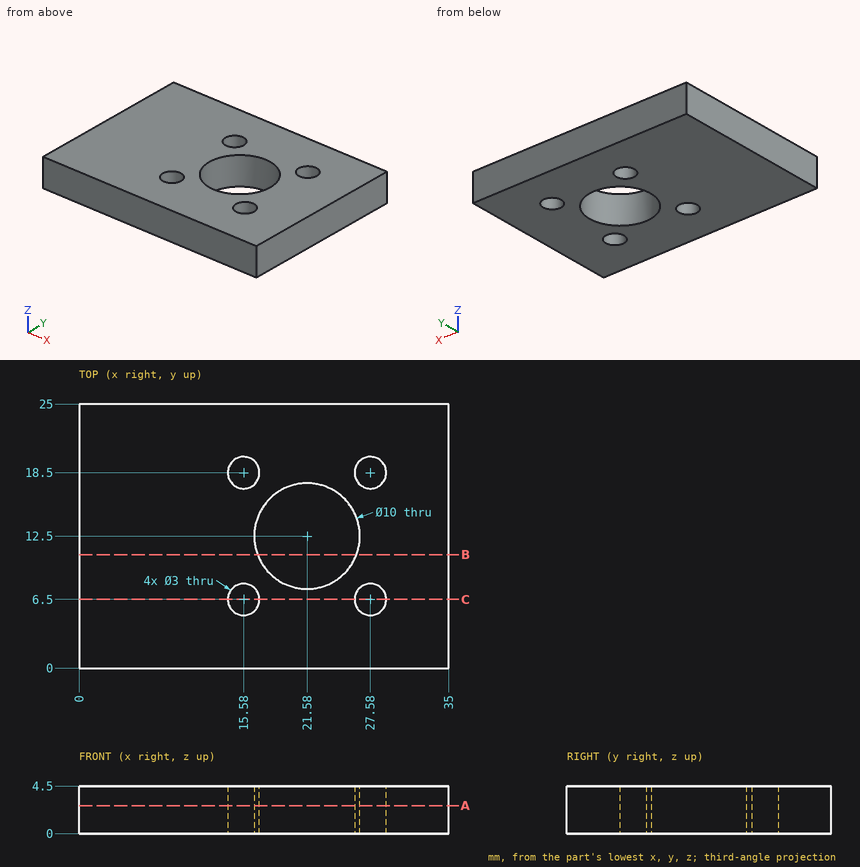
Design review of the part shown in the three views and the two pictorial views. Dimensions are in mm from the part's minimum x, y and z. Coordinates: 2 decimals unless noted, no trailing zeros. Order: outer loops, then holes, each group sorted by start corner. A loop starts at its lowest first (then second) coordinate and runs counter-clockwise, first axis right, second up.
1) Clearance check with a flat-ended pin moving along its axis: pin 1 (1 mm diameter, centred on x = 6.5, z = 3, fed in from -Y). State where the tip first meets the part, or that it passes through.
2) Wall thickness on line 1 along Y through (x, z) = (27.5, 2.7); line 2 along X through (y, z) = (5.25, 0.8); line 3 along X through (y, z) = (21.75, 3.35) (1 decimal): over which ranges is each line inside the solid? List them lowest first.
3) Take a section at B-B, the plane y = 10.75. Give the boundary of the cut face in (x, z), and give its area (3 significant figures).
4) Take a section at C-C, the plane y = 6.5. Give the boundary of the cut face in (x, z).
5) Take a section at A-A, the plane z = 2.65. Give the boundary of the cut face in (x, y) (1 decimal), and give its area (3 significant figures).
Returned:
1. pin 1: stops at y = 0.01
2. line 1: y = 0 to 5, 8 to 17, 20 to 25
2. line 2: x = 0 to 14.75, 16.41 to 26.75, 28.41 to 35
2. line 3: x = 0 to 35
3. outline: (0, 0) - (16.9, 0) - (16.9, 4.5) - (0, 4.5) - close; (26.26, 0) - (35, 0) - (35, 4.5) - (26.26, 4.5) - close
3. area: 115 mm2
4. outline: (0, 0) - (14.08, 0) - (14.08, 4.5) - (0, 4.5) - close; (17.08, 0) - (26.08, 0) - (26.08, 4.5) - (17.08, 4.5) - close; (29.08, 0) - (35, 0) - (35, 4.5) - (29.08, 4.5) - close
5. outline: (0, 0) - (35, 0) - (35, 25) - (0, 25) - close; hole circle Ø3 at (15.6, 6.5); hole circle Ø3 at (15.6, 18.5); hole circle Ø10 at (21.6, 12.5); hole circle Ø3 at (27.6, 6.5); hole circle Ø3 at (27.6, 18.5)
5. area: 768 mm2
